Source: CAD feature listing. Evaluate the final solid. Frame: model axes, mm. Face numbers are marked on the shaded views. A direction names the side the tool comes from. Round coordinates to 2 decimals unless told otherwise and drop trailing zeros. Loops run counter-clockwise (first coordinate to the right, second up) from the corner with the lowest first, then second, coordinate; pieces in that order, holes last. Notation, with made-up numbers: M 47,76 L 100,76 A23 cw 100,99 Z; hole C -34,49.5 d10. An arc over 180 degrees is marked long. One line per item, written item: value.
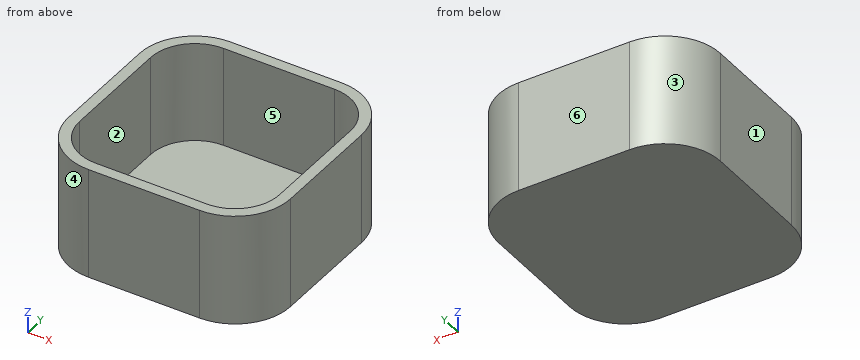
from build123d import *

# Parameters (mm, degrees)
F0_W     = 40
F0_H     = 40
F1_DEPTH = 20
F2_R     = 10
F3_T     = -2


with BuildPart() as f1:
    # F0 (on Top) → F1 (new body)
    with BuildSketch(Plane.XY):
        Rectangle(F0_W, F0_H)
    extrude(amount=-F1_DEPTH)

    # F2
    f2_edges = [f1.edges().sort_by_distance(p)[0] for p in [
        (-20, -20, -10),
        (20, -20, -10),
        (20, 20, -10),
        (-20, 20, -10),
    ]]
    fillet(f2_edges, radius=F2_R)

    # F3
    f3_openings = [f1.faces().sort_by_distance(p)[0] for p in [
        (0, 0, 0),
    ]]
    offset(amount=F3_T, openings=f3_openings)


solid = f1.part
1. Reachability of the marked faces 5 and 6 from +Z, -Z, +X, -X, +Y, -Y: full face, straight path, thin tool, end or side. Return the list, or none.
Report:
face 5: +Z
face 6: +Z, -Z, +X, -X, +Y
2. Section query B-B (x = -8). Return the cut outline in (y, z), and give its area (3 significant figures).
Report:
outline: M -20,-20 L 20,-20 L 20,0 L 18,0 L 18,-18 L -18,-18 L -18,0 L -20,0 Z
area: 152 mm2
3. Pin query (flat end, axial travel): pin 1 (4 mm diameter, centred on x = 8.5, y = 10, fed in from +Z); pin 2 (6 mm diameter, centred on y = -15, z = -13, fed in from +X). Return the tip coordinate at first contact, or that it passes through.
Report:
pin 1: stops at z = -18
pin 2: stops at x = 19.8
4. Ray query, line 1 (Y direction, x = -1, z = -16.75); line 2 (Z direction, x = 12, y = -7). Return the intervals inside material, ascending. Write a range as [from, to].
Report:
line 1: y = [-20, -18], [18, 20]
line 2: z = [-20, -18]
5. Section query A-A (z = -10.5). Return the cut outline in (x, y), and give its area (3 significant figures).
Report:
outline: M -20,-10 A10 ccw -10,-20 L 10,-20 A10 ccw 20,-10 L 20,10 A10 ccw 10,20 L -10,20 A10 ccw -20,10 Z; hole M -18,-10 A8 ccw -10,-18 L 10,-18 A8 ccw 18,-10 L 18,10 A8 ccw 10,18 L -10,18 A8 ccw -18,10 Z
area: 273 mm2
6. Pull-direction query (Y, two-part tool) for the marked faces 1, 2, 3 and 4; classes: released by +Y, released by -Y, zero draft, split by the parting line, or undercut.
Report:
face 1: zero draft
face 2: undercut
face 3: released by +Y
face 4: released by -Y
